Autodesk Inventor part; units mm, degrees
ref_plane "YZ Plane" through (0, 0, 0) normal (1, 0, 0) x (0, 1, 0)
ref_plane "XZ Plane" through (0, 0, 0) normal (0, 1, 0) x (-1, 0, 0)
ref_plane "XY Plane" through (0, 0, 0) normal (0, 0, 1) x (1, 0, 0)
sketch "Sketch1" plane through (0, 0, 0) normal (0, 1, 0) x (-1, 0, 0)
  line L0 (0, 0) -> (8.89, 0)
  line L1 (8.89, 0) -> (8.89, -16.002)
  line L2 (8.89, -16.002) -> (0, -16.002)
  line L3 (0, -16.002) -> (0, 0)
  dimension "d0" = 8.89
  dimension "d1" = 16.002
extrude "Extrusion1" add sketch "Sketch1" along normal blind 2.54
sketch "Sketch5" plane through (0, 2.54, 0) normal (0, 1, 0) x (1, 0, 0)
  line L0 (-8.89, 0) -> (0, 0)
  line L1 (0, 0) -> (0, 16.002)
  line L2 (0, 16.002) -> (-8.89, 16.002)
  line L3 (-8.89, 16.002) -> (-8.89, 0)
  line L4 (0, 0) -> (-8.89, 0)
  line L5 (-5.842, 0) -> (-6.731, 1.016)
  line L6 (-6.731, 1.016) -> (-6.731, 1.778)
  line L7 (-6.731, 1.778) -> (-2.159, 1.778)
  line L8 (-2.159, 1.778) -> (-2.159, 1.016)
  line L9 (-2.159, 1.016) -> (-3.048, 0)
  line L10 (-8.89, 0) -> (-8.89, 16.002)
  line L11 (-8.89, 3.81) -> (0, 3.81)
  point P0 (-4.445, 1.778)
  point P1 (-4.445, 3.81)
  dimension "d19" = 2.794
  dimension "d20" = 4.572
  dimension "d21" = 1.016
  dimension "d23" = 1.778
  dimension "d24" = 3.81
extrude "Extrusion4" add sketch "Sketch5" along normal blind 1.27 contours L3 L11 L1 L0 L9 L8 L7 L6 L5
sketch "Sketch6" plane through (0, 2.54, 0) normal (0, 1, 0) x (1, 0, 0)
  line L0 (-3.048, 0) -> (-2.159, 1.016)
  line L1 (-2.159, 1.016) -> (-2.159, 1.778)
  line L2 (-2.159, 1.778) -> (-6.731, 1.778)
  line L3 (-6.731, 1.778) -> (-6.731, 1.016)
  line L4 (-6.731, 1.016) -> (-5.842, 0)
  line L5 (-5.842, 0) -> (-3.048, 0)
  point P0 (0, 0)
extrude "Extrusion5" cut sketch "Sketch6" against normal blind 2.032
fillet "Fillet3" radius 1.27 6 edges at (-8.89, 1.27, -16.002) (0, 1.27, -16.002) (-8.89, 1.905, 0) (-8.89, 3.175, -3.81) (0, 3.175, -3.81) (0, 1.905, 0)
sketch "Sketch8" plane through (0, 2.54, 0) normal (0, 1, 0) x (1, 0, 0)
  line L0 (-7.62, 16.002) -> (-1.27, 16.002)
  line L1 (-6.1595, 16.002) -> (-6.1595, 11.557)
  line L2 (-2.7305, 16.002) -> (-2.7305, 11.557)
  arc A0 (-6.1595, 11.557) -> (-2.7305, 11.557) centre (-4.445, 11.557) ccw
  point P0 (0, 0)
  point P1 (-4.445, 16.002)
  dimension "d37" = 3.429
  dimension "d38" = 4.445
extrude "Extrusion7" cut sketch "Sketch8" against normal blind 25.4
fillet "Fillet4" radius 1.016 2 edges at (-2.7305, 1.27, -16.002) (-6.1595, 1.27, -16.002)
properties part number "HallEffectSpoolSensorMount3" material "ABS Plastic"
Verification items for the finished model (mm, model axes). A direction names the side the tool comes from. Round coordinates to 2 decimals unless told otherwise and drop trailing zeros. Write each loop counter-clockwise with the first axis right and the second up, starting at its lowest first coordinate (ties: lowest second). Pieces come first, ordered by that corner, then holes.
1. Section check B-B on y = 2.05. Enter the section's corners in (x, z) (1 decimal), plus the area to 3 significant figures.
2. Section check D-D on z = -10.75. Enter the section's corners in (x, y), plus the area to 3 significant figures.
3. Access from +Z, -Z, +X, -X, +Y, -Y to the whole of each face (thin tool, end or side, straight path). Record for faces 1 (the flat face through (-4, 0.508, -1)), 2 (the flat face through (-6.16, 1, -13)), 3 (the cylindrical face through (-8.508, 3.184, -3.448)).
4. Section check C-C on x = -3.5. Enter the section's corners in (y, z), plus the area to 3 significant figures.
5. Gauge pin test, flat ends, axial feed: P1, Ø1.4, axis at x = -4.5, y = 3.5, coming from the -Z side; P2, Ø1, axis at x = -4, y = 2, coming from the +Z side. Record the tip position at first contact, or that the pin passes through.
6. Section check A-A on z = -14.5. Enter the section's corners in (x, y), plus the area to 3 significant figures.
7. Scan lines: L1, parallel to X at y = 0.7, z = -13.25; L2, parallel to Y at x = -5.5, z = -9.75; L3, parallel to Z at x = -4, y = 2.8. Record each from-to range of solid material in increasing order.
Answer:
1. outline: (-8.9, -14.7) arc R1.3 ccw to (-7.6, -16) - (-7.2, -16) arc R1 ccw to (-6.2, -15) - (-6.2, -11.6) arc R1.7 cw to (-2.7, -11.6) - (-2.7, -15) arc R1 ccw to (-1.7, -16) - (-1.3, -16) arc R1.3 ccw to (0, -14.7) - (0, -1.3) arc R1.3 ccw to (-1.3, 0) - (-3, 0) - (-2.2, -1) - (-2.2, -1.8) - (-6.7, -1.8) - (-6.7, -1) - (-5.8, 0) - (-7.6, 0) arc R1.3 ccw to (-8.9, -1.3) - close
1. area: 113 mm2
2. outline: (-8.89, 0) - (-5.96, 0) - (-5.96, 2.54) - (-8.89, 2.54) - close; (-2.93, 0) - (0, 0) - (0, 2.54) - (-2.93, 2.54) - close
2. area: 14.9 mm2
3. face 1: +Y
3. face 2: -Z, +Y, -Y
3. face 3: -Z, -X, +Y
4. outline: (0, -10.13) - (2.54, -10.13) - (2.54, -3.81) - (3.81, -3.81) - (3.81, -1.78) - (0.51, -1.78) - (0.51, 0) - (0, 0) - close
4. area: 24.7 mm2
5. P1: stops at z = -3.81
5. P2: stops at z = -1.78
6. outline: (-8.89, 0) - (-6.16, 0) - (-6.16, 2.54) - (-8.89, 2.54) - close; (-2.73, 0) - (0, 0) - (0, 2.54) - (-2.73, 2.54) - close
6. area: 13.9 mm2
7. L1: x = -8.89 to -6.16, -2.73 to 0
7. L2: y = 0 to 2.54
7. L3: z = -3.81 to -1.78
